Here's how the part is built. I have some questions about the finished solid (model axes, mm). Face numbers are marked on the shaded views. A direction names the side the tool comes from. Coordinates: 2 decimals unless noted, no trailing zeros. Order: outer loops, then holes, each group sorted by start corner. A loop starts at its lowest first (then second) coordinate and runs counter-clockwise, first axis right, second up. Notation, with made-up numbers: (85.25, 84) - (138.25, 84) arc R10 ccw to (138.25, 97) - close; hole circle Ø7 at (44, -7). An arc over 180 degrees is marked (long way). Answer in a Markdown table with one row per item. Add a question column.
Item 1: I want a section at A-A (x = 86.5). Please give me the cut outline in (y, z).
Item 2: I want a section at B-B (y = 4). Please give me the cut outline in (x, z).
Item 3: If I drill on line 1 along Z through (x, y) = (3.75, 160); line 2 along Y through (x, z) = (5, 5); line 3 along Y through (x, z) = (91.5, 21), over which ranges is the centre line in solid material (lowest first)? Write a range as from..to.
Item 4: I want a section at D-D (x = 48.5). Please give me the cut outline in (y, z).
Item 5: Thinking about a two-plate mould opening in Y: for the marked faces 4, 5 and 6, which applies, +Y half, -Y half, draft (parallel to the pull), parting line (faces both ways), or undercut?
Item 6: On a 3-axis mill with a long thin cutter (end or side, diameter ignored), from which of +Z, -Z, +X, -X, +Y, -Y can I reach the whole of each face in a straight line? I mean the marked faces 1, 2 and 3. Say none if no direction works.
Item 7: I want a section at C-C (y = 86). Please give me the cut outline in (x, z).
Item 8: Will these pins go through, and if not, where does the flat tip stop? pin 1 Ø5 at (y, z) = (45, 19) entering from -X; pin 2 Ø1 at (y, z) = (154, 63) entering from +X; pin 3 Ø1 at (x, z) = (60.5, 53.5) entering from -Y; pin 4 Ø10 at (x, y) = (103.5, 95.5) entering from -Z.
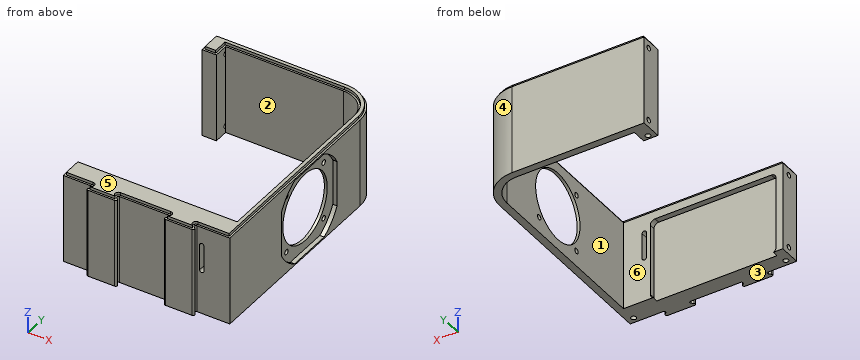
Autodesk Inventor part; units mm, degrees
ref_plane "YZ Plane" through (0, 0, 0) normal (1, 0, 0) x (0, 1, 0)
ref_plane "XZ Plane" through (0, 0, 0) normal (0, 1, 0) x (-1, 0, 0)
ref_plane "XY Plane" through (0, 0, 0) normal (0, 0, 1) x (1, 0, 0)
sketch "Sketch1" plane through (0, 0, 0) normal (0, 0, 1) x (1, 0, 0)
  line L0 (0, 0) -> (116, 0)
  line L1 (116, 0) -> (116, 141)
  arc A0 (116, 141) -> (92, 165) centre (92, 141) ccw
  line L2 (0, 0) -> (0, 165)
  line L3 (0, 165) -> (92, 165)
  dimension "d0" = 24
  dimension "d1" = 92
  dimension "d2" = 165
extrude "Extrusion1" add sketch "Sketch1" along normal blind 62
shell "Shell2" thickness 5 removed faces 3 at (0, 110, 20.6667) at (38.6667, 102, 0) at (38.6667, 102, 62)
sketch "Sketch6" plane through (0, 160, 0) normal (0, -1, 0) x (1, 0, 0)
  line L0 (0, 0) -> (10, 0)
  line L1 (10, 0) -> (10, 10)
  line L2 (10, 10) -> (0, 10)
  line L3 (0, 10) -> (0, 0)
  dimension "d90" = 2
  dimension "d91" = 0
  dimension "d38" = 10
  dimension "d39" = 10
sketch "Sketch7" plane through (0, 160, 0) normal (0, -1, 0) x (1, 0, 0)
  line L0 (0, 62) -> (10, 62)
  line L1 (10, 62) -> (10, 52)
  line L2 (10, 52) -> (0, 52)
  line L3 (0, 52) -> (0, 62)
  line L4 (92, 0) -> (0, 0)
  line L5 (92, 0) -> (92, 62)
  line L6 (0, 62) -> (92, 62)
  line L7 (0, 0) -> (0, 62)
  point P0 (0, 0)
  dimension "d40" = 10
  dimension "d41" = 10
extrude "Extrusion6" add sketch "Sketch6" along normal blind 10
extrude "Extrusion7" add sketch "Sketch7" along normal blind 10 contours L0 L1 L2 L3
sketch "Sketch9" plane through (0, 5, 0) normal (0, 1, 0) x (1, 0, 0)
  line L0 (0, 0) -> (111, 0)
  line L1 (0, -62) -> (0, 0)
  line L2 (111, -62) -> (0, -62)
  line L3 (111, 0) -> (111, -62)
extrude "Extrusion8" add sketch "Sketch9" along normal blind 10
sketch "Sketch10" plane through (0, 15, 0) normal (0, 1, 0) x (1, 0, 0)
  arc A0 (5, -53) -> (8, -56) centre (8, -53) ccw
  arc A1 (8, 0) -> (5, -3) centre (8, -3) ccw
  line L0 (5, -53) -> (5, -3)
  arc A2 (92, -3) -> (89, 0) centre (89, -3) ccw
  arc A3 (89, -56) -> (92, -53) centre (89, -53) ccw
  line L1 (89, -56) -> (8, -56)
  line L2 (89, 0) -> (8, 0)
  line L3 (92, -53) -> (92, -3)
  line L4 (0, 0) -> (0, -62)
  line L5 (111, 0) -> (0, 0)
  arc A4 (4.7, -53) -> (8, -56.3) centre (8, -53) ccw
  line L6 (4.7, -53) -> (4.7, -3)
  arc A5 (8, 0.3) -> (4.7, -3) centre (8, -3) ccw
  line L7 (8, 0.3) -> (89, 0.3)
  arc A6 (92.3, -3) -> (89, 0.3) centre (89, -3) ccw
  line L8 (92.3, -3) -> (92.3, -53)
  arc A7 (89, -56.3) -> (92.3, -53) centre (89, -53) ccw
  line L9 (89, -56.3) -> (8, -56.3)
  point P0 (6.6252, 0)
  point P1 (90.3748, 0)
  point P2 (89, 0)
  dimension "d48" = 81
  dimension "d49" = 3
  dimension "d50" = 50
  dimension "d51" = 3
  dimension "d52" = 81
  dimension "d53" = 3
  dimension "d54" = 50
  dimension "d55" = 3
  dimension "d56" = 5
  dimension "d57" = 0.3
extrude "Extrusion9" cut sketch "Sketch10" against normal blind 4 contours L0 A1 L2 A2 L3 A3 L1 A0 | A0 L1 A3 L3 A2 L5 A6 L8 A7 L9 A4 L6 A5 A1 L0
sketch "Sketch12" plane through (0, 160, 10) normal (0, 0, 1) x (1, 0, 0)
  line L0 (0, 0) -> (10, 0)
  line L1 (0, 0) -> (0, -10)
  line L2 (10, -10) -> (0, -10)
  line L3 (10, 0) -> (10, -10)
  point P0 (0, -160)
extrude "Extrusion11" add sketch "Sketch12" along normal up to surface (42 mm away)
sketch "Sketch14" plane through (0, 0, 62) normal (0, 0, 1) x (1, 0, 0)
  line L0 (36.5757, 0) -> (41.5757, -5)
  line L1 (22, 0) -> (37, 0)
  line L2 (17.3, -4.7) -> (41.7, -4.7)
  line L3 (22.4243, 0) -> (17.4243, -5)
  line L4 (22, 0) -> (17, -5)
  line L5 (-3, 0) -> (-3, -5)
  line L6 (96, -5) -> (91, 0)
  line L7 (42, -5) -> (37, 0)
  line L8 (71, -5) -> (76, 0)
  line L9 (76.4243, 0) -> (71.4243, -5)
  line L10 (76, 0) -> (91, 0)
  line L11 (71.3, -4.7) -> (95.7, -4.7)
  line L12 (116, 0) -> (-3, 0)
  line L13 (-3, 0) -> (116, 0)
  line L14 (-3, -5) -> (116, -5)
  line L15 (90.5757, 0) -> (95.5757, -5)
  line L16 (116, 0) -> (116, -5)
  line L17 (10, 160) -> (92, 160)
  arc A0 (111, 141) -> (92, 160) centre (92, 141) ccw
  line L18 (111, 141) -> (111, 15)
  line L19 (0, 15) -> (111, 15)
  line L20 (0, 15) -> (0, 0)
  line L21 (0, 0) -> (116, 0)
  line L22 (116, 0) -> (116, 141)
  arc A1 (116, 141) -> (92, 165) centre (92, 141) ccw
  line L23 (92, 165) -> (0, 165)
  line L24 (0, 165) -> (0, 150)
  line L25 (10, 150) -> (0, 150)
  line L26 (10, 160) -> (10, 150)
  point P0 (95.2757, -4.7)
  point P1 (71.7243, -4.7)
  point P2 (17.7243, -4.7)
  point P3 (41.2757, -4.7)
  dimension "d70" = 5
  dimension "d71" = 45
  dimension "d72" = 45
  dimension "d73" = 45
  dimension "d74" = 20
  dimension "d75" = 25
  dimension "d76" = 25
  dimension "d77" = 20
  dimension "d78" = 119
  dimension "d79" = 0.3
  dimension "d80" = 0.3
  dimension "d81" = 0.3
  dimension "d82" = 0.3
  dimension "d83" = 0.3
  dimension "d84" = 0.3
extrude "Extrusion12" add sketch "Sketch14" against normal up to surface (62 mm away) contours L0 L2 L3 L1 | L10 L15 L11 L9
fillet "Fillet4" radius 1 8 edges at (22.4243, 0, 31) (17.7243, -4.7, 31) (41.2757, -4.7, 31) (76.4243, 0, 31) (71.7243, -4.7, 31) (95.2757, -4.7, 31) (36.5757, 0, 31) (90.5757, 0, 31)
sketch "Sketch15" plane through (0, 0, 62) normal (0, 0, 1) x (1, 0, 0)
  arc A0 (92.8615, -4.7) -> (93.5686, -2.9929) centre (92.8615, -3.7) ccw
  line L0 (93.5686, -2.9929) -> (92.2828, -1.7071)
  arc A1 (92.9899, 0) -> (92.2828, -1.7071) centre (92.9899, -1) ccw
  line L1 (92.9899, 0) -> (116, 0)
  line L2 (116, 0) -> (116, 141)
  arc A2 (116, 141) -> (92, 165) centre (92, 141) ccw
  line L3 (92, 165) -> (0, 165)
  line L4 (0, 165) -> (0, 150)
  line L5 (10, 150) -> (0, 150)
  line L6 (10, 160) -> (10, 150)
  line L7 (10, 160) -> (92, 160)
  arc A3 (111, 141) -> (92, 160) centre (92, 141) ccw
  line L8 (111, 141) -> (111, 15)
  line L9 (0, 15) -> (111, 15)
  line L10 (0, 15) -> (0, 0)
  line L11 (0, 0) -> (20.0101, 0)
  arc A4 (20.7172, -1.7071) -> (20.0101, 0) centre (20.0101, -1) ccw
  line L12 (20.7172, -1.7071) -> (19.4314, -2.9929)
  arc A5 (19.4314, -2.9929) -> (20.1385, -4.7) centre (20.1385, -3.7) ccw
  line L13 (20.1385, -4.7) -> (38.8615, -4.7)
  arc A6 (38.8615, -4.7) -> (39.5686, -2.9929) centre (38.8615, -3.7) ccw
  line L14 (39.5686, -2.9929) -> (38.2828, -1.7071)
  arc A7 (38.9899, 0) -> (38.2828, -1.7071) centre (38.9899, -1) ccw
  line L15 (38.9899, 0) -> (74.0101, 0)
  arc A8 (74.7172, -1.7071) -> (74.0101, 0) centre (74.0101, -1) ccw
  line L16 (74.7172, -1.7071) -> (73.4314, -2.9929)
  arc A9 (73.4314, -2.9929) -> (74.1385, -4.7) centre (74.1385, -3.7) ccw
  line L17 (74.1385, -4.7) -> (92.8615, -4.7)
  line L18 (112.3, 13.7) -> (112.3, 141)
  arc A10 (112.3, 141) -> (92, 161.3) centre (92, 141) ccw
  line L19 (92, 161.3) -> (8.7, 161.3)
  line L20 (8.7, 161.3) -> (8.7, 151.3)
  line L21 (8.7, 151.3) -> (1.3, 151.3)
  line L22 (1.3, 151.3) -> (1.3, 163.7)
  line L23 (1.3, 163.7) -> (92, 163.7)
  arc A11 (114.7, 141) -> (92, 163.7) centre (92, 141) ccw
  line L24 (114.7, 141) -> (114.7, 1.3)
  line L25 (114.7, 1.3) -> (92.9899, 1.3)
  arc A12 (92.9899, 1.3) -> (91.3636, -2.6263) centre (92.9899, -1) ccw
  line L26 (91.3636, -2.6263) -> (92.1373, -3.4)
  line L27 (92.1373, -3.4) -> (74.8627, -3.4)
  line L28 (74.8627, -3.4) -> (75.6364, -2.6263)
  arc A13 (75.6364, -2.6263) -> (74.0101, 1.3) centre (74.0101, -1) ccw
  line L29 (74.0101, 1.3) -> (38.9899, 1.3)
  arc A14 (38.9899, 1.3) -> (37.3636, -2.6263) centre (38.9899, -1) ccw
  line L30 (37.3636, -2.6263) -> (38.1373, -3.4)
  line L31 (38.1373, -3.4) -> (20.8627, -3.4)
  line L32 (20.8627, -3.4) -> (21.6364, -2.6263)
  arc A15 (21.6364, -2.6263) -> (20.0101, 1.3) centre (20.0101, -1) ccw
  line L33 (20.0101, 1.3) -> (1.3, 1.3)
  line L34 (1.3, 1.3) -> (1.3, 13.7)
  line L35 (1.3, 13.7) -> (112.3, 13.7)
  dimension "d89" = 1.3
extrude "Extrusion13" add sketch "Sketch15" along normal blind 2 contours L18 A10 L19 L20 L21 L22 L23 A11 L24 L25 A12 L26 L27 L28 A13 L29 A14 L30 L31 L32 A15 L33 L34 L35
sketch "Sketch16" plane through (0, 15, 0) normal (0, 1, 0) x (1, 0, 0)
  line L0 (96.5, -31) -> (96.5, -49) construction
  line L1 (95, -31) -> (95, -49)
  line L2 (98, -49) -> (98, -31)
  arc A0 (98, -31) -> (95, -31) centre (96.5, -31) ccw
  arc A1 (95, -49) -> (98, -49) centre (96.5, -49) ccw
  line L3 (92.3, -3) -> (92.3, -53)
  line L4 (0, -62) -> (111, -62)
  line L5 (116, 0) -> (116, -62)
  line L6 (116, 0) -> (116, -62)
  point P0 (0, 0)
  point P1 (96.5, -40)
  point P2 (116, -31)
  dimension "d92" = 18
  dimension "d93" = 3
  dimension "d95" = 13
  dimension "d98" = 18
extrude "Extrusion14" cut sketch "Sketch16" against normal through all
sketch "Sketch17" plane through (116, 0, 0) normal (1, 0, 0) x (0, 0, -1)
  circle A0 centre (-51.1525, 65.8475) radius 1.8
  arc A1 (-61, 70) -> (-47, 56) centre (-31, 86) ccw
  line L0 (4, 51) -> (-66, 51)
  line L1 (-61, 56) -> (-1, 56) construction
  line L2 (-15, 56) -> (-47, 56)
  circle A2 centre (-10.8475, 65.8475) radius 1.8
  arc A3 (-15, 56) -> (-1, 70) centre (-31, 86) ccw
  line L3 (-1, 102) -> (-1, 70)
  circle A4 centre (-10.8475, 106.1525) radius 4 construction
  circle A5 centre (-10.8475, 106.1525) radius 1.8
  arc A6 (-1, 102) -> (-15, 116) centre (-31, 86) ccw
  line L4 (-61, 70) -> (-61, 102)
  line L5 (-61, 116) -> (-61, 56) construction
  arc A7 (-47, 116) -> (-61, 102) centre (-31, 86) ccw
  line L6 (-66, 51) -> (-66, 121)
  line L7 (-47, 116) -> (-15, 116)
  circle A8 centre (-31, 86) radius 23.5 construction
  circle A9 centre (-31, 86) radius 24
  line L8 (-1, 116) -> (-61, 56) construction
  line L9 (-61, 116) -> (-1, 56) construction
  line L10 (-1, 56) -> (-1, 116) construction
  line L11 (4, 121) -> (4, 51)
  circle A10 centre (-31, 86) radius 34 construction
  line L12 (4, 121) -> (-66, 51) construction
  line L13 (-66, 121) -> (4, 51) construction
  line L14 (-1, 116) -> (-61, 116) construction
  line L15 (-66, 121) -> (4, 121)
  circle A11 centre (-51.1525, 106.1525) radius 1.8
  line L16 (0, 0) -> (0, 141)
  line L17 (0, 141) -> (-62, 141)
  point P0 (-1, 102)
  point P1 (-47, 56)
  point P2 (-1, 70)
  point P3 (-15, 116)
  dimension "d101" = 60
  dimension "d102" = 60
  dimension "d103" = 68
  dimension "d104" = 47
  dimension "d105" = 8
  dimension "d106" = 28.5
  dimension "d107" = 3.6
  dimension "d108" = 48
  dimension "d109" = 360
  dimension "d110" = 70
  dimension "d111" = 70
  dimension "d114" = 20
  dimension "d119" = 1
extrude "Extrusion15" cut sketch "Sketch17" against normal blind 3 contours L4 A7 L7 A6 L3 A3 L2 A1
extrude "Extrusion16" cut sketch "Sketch17" against normal through all contours A0 | A2 | A5 | A9 | A11
sketch "Sketch18" plane through (0, 0, 0) normal (0, 0, -1) x (-1, 0, 0)
  circle A0 centre (-5, 153) radius 1.8
  line L0 (0, 150) -> (-10, 150)
  line L1 (-10, 160) -> (-10, 150)
  circle A1 centre (-111, 4) radius 1.8
  circle A2 centre (-5, 4) radius 1.8
  line L2 (-6.6252, 15) -> (0, 15)
  line L3 (0, 0) -> (-20.0101, 0)
  line L4 (-92.9899, 0) -> (-116, 0)
  line L5 (-116, 0) -> (-116, 141)
  line L6 (0, 15) -> (0, 0)
  dimension "d120" = 3.6
  dimension "d121" = 3
  dimension "d122" = 5
  dimension "d123" = 10
  dimension "d124" = 3.6
  dimension "d125" = 3.6
  dimension "d126" = 15
  dimension "d127" = 4
  dimension "d128" = 4
  dimension "d129" = 5
  dimension "d130" = 5
extrude "Extrusion17" cut sketch "Sketch18" against normal blind 10
sketch "Sketch19" plane through (0, 165, 0) normal (-1, 0, 0) x (0, 0, 1)
  line L0 (10, -13.8) -> (10, -10.2)
  line L1 (0, -13.8) -> (0, -10.2)
  circle A0 centre (5, -5) radius 1.8
  circle A1 centre (57, -5) radius 1.8
  circle A2 centre (5, -156.5) radius 1.8
  circle A3 centre (57, -156.5) radius 1.8
  line L2 (0, -5) -> (62.0541, -5) construction
  line L3 (0, 0) -> (62, 0) construction
  line L4 (62, 0) -> (62, -15) construction
  line L5 (0, 0) -> (0, -15) construction
  line L6 (62, -150) -> (62, -165) construction
  line L7 (0, -150) -> (62, -150) construction
  line L8 (0, -150) -> (0, -165) construction
  dimension "d133" = 3.6
  dimension "d134" = 3.6
  dimension "d135" = 3.6
  dimension "d136" = 3.6
  dimension "d137" = 5
  dimension "d138" = 5
  dimension "d139" = 5
  dimension "d140" = 5
  dimension "d141" = 5
  dimension "d142" = 6.5
  dimension "d143" = 5
  dimension "d144" = 6.5
extrude "Extrusion18" cut sketch "Sketch19" against normal blind 10
properties part number "ElecTweetBox"
Values follow:
| question | item | result |
|---|---|---|
| 1 | outline | (-4.7, 0) - (11, 0) - (11, 56.3) - (15, 56.3) - (15, 62) - (13.7, 62) - (13.7, 64) - (-3.4, 64) - (-3.4, 62) - (-4.7, 62) - close; (160, 0) - (165, 0) - (165, 62) - (163.7, 62) - (163.7, 64) - (161.3, 64) - (161.3, 62) - (160, 62) - close |
| 2 | outline | (0, 0) - (3.2, 0) - (3.2, 10) - (6.8, 10) - (6.8, 0) - (109.2, 0) - (109.2, 10) - (112.8, 10) - (112.8, 0) - (116, 0) - (116, 62) - (114.7, 62) - (114.7, 64) - (1.3, 64) - (1.3, 62) - (0, 62) - close; hole (95, 31) arc R1.5 ccw to (98, 31) - (98, 49) arc R1.5 ccw to (95, 49) - close |
| 3 | line 1 | z = 0..3.2, 6.8..55.2, 58.8..64 |
| 3 | line 2 | y = 0..2.2, 5.8..6.7, 10.3..11, 150..151.2, 154.8..158.2, 161.8..165 |
| 3 | line 3 | y = -4.7..11, 160..165 |
| 4 | outline | (0, 0) - (11, 0) - (11, 56.3) - (15, 56.3) - (15, 62) - (13.7, 62) - (13.7, 64) - (1.3, 64) - (1.3, 62) - (0, 62) - close; (160, 0) - (165, 0) - (165, 62) - (163.7, 62) - (163.7, 64) - (161.3, 64) - (161.3, 62) - (160, 62) - close |
| 5 | face 4 | +Y half |
| 5 | face 5 | draft |
| 5 | face 6 | undercut |
| 6 | face 1 | +Z, -Z, -X |
| 6 | face 2 | +Z, -Z |
| 6 | face 3 | -Z, +X, -X, +Y, -Y |
| 7 | outline | (111, 0) - (116, 0) - (116, 1) - (113, 1) - (113, 7) - (111, 7) - close; (111, 55) - (113, 55) - (113, 61) - (116, 61) - (116, 62) - (114.7, 62) - (114.7, 64) - (112.3, 64) - (112.3, 62) - (111, 62) - close |
| 8 | pin 1 | stops at x = 111 |
| 8 | pin 2 | stops at x = 110.95 |
| 8 | pin 3 | stops at y = 0 |
| 8 | pin 4 | passes through |
